Design review of the part built by this model. Coordinates are the model's own, in mm. Round coordinates to 2 decimals unless told otherwise and drop trailing zeros. Order: outer loops, then holes, each group sorted by start corner. A loop starts at its lowest first (then second) coordinate and runs counter-clockwise, first axis right, second up. Notation, with made-up numbers: M 14,33 L 64,33 A38 cw 64,72 Z; hole C -37,-36 d8. An arc over 180 degrees is marked long. Use a Markdown table: item, result. Add a question column.
(1) Take a section at B-B (z = -36.5). Write out the cut boundary in (x, y).
(2) For pin 1 (1.5 mm diameter, centred on y = -1, z = 7, fed in from +X); pin 2 (23 mm diameter, centred on x = 75.01, z = 0, fed in from -Y); pin 3 (2 mm diameter, centred on y = -3, z = -19, fed in from -X), all flat-tipped, find the tip position at first contact; note any pin that passes through.
(3) The part is to be moulded in two halves that separate along X. For faces 1 (the face through (-64.086, -3.131, 3.815)), 2 (the face through (1.22, -3.13, 63.49)), 3 (the face through (45, 0, 1)), say which applies: released by +X, released by -X, zero draft, split by the parting line, or undercut.
(4) Take a section at A-A (x = 85). Write out the cut boundary in (y, z).
(5) Take a section at C-C (z = 9). Write out the cut boundary in (x, y).
(6) To check wall thickness, follow probe 1 along Z at (x, y) = (0, -2.5); probe 2 along X at (y, z) = (-4.25, 4); probe 3 along Z at (x, y) = (74.5, -1.25). State the ranges of each line that lie inside material, in increasing order. Write a range as from..to.
(7) Take a section at D-D (y = -2). Write out the cut boundary in (x, z).
```python
from build123d import *

# Parameters (mm, degrees)
F0_R     = 12.7
F1_DEPTH = 6.35


# Not quite as in the source:
# - a length typed as a fraction of an inch, garbled in the dataset ("3 / 203.2 mm" for 3/8 in), is restored


with BuildPart() as f1:
    # F0 (on Front) → F1 (new body)
    with BuildSketch(Plane.XZ):
        with BuildLine():
            ThreePointArc((-46.13671875, -43.6308741946), (-24.8918341596, -58.4178619274), (0.4890866537, -63.4981164622))
            ThreePointArc((0.4890866537, -63.4981164622), (25.7887406506, -58.0275008566), (46.8033281156, -42.9150145905))
            ThreePointArc((46.8033281156, -42.9150145905), (59.5789989506, -33.7738186545), (74.9568035052, -30.5640903944))
            ThreePointArc((74.9568035052, -30.5640903944), (105.5782883644, 0), (74.9568035052, 30.5640903944))
            ThreePointArc((74.9568035052, 30.5640903944), (59.5789989506, 33.7738186545), (46.8033281156, 42.9150145905))
            ThreePointArc((46.8033281156, 42.9150145905), (0.4890866537, 63.4981164622), (-46.13671875, 43.6308741946))
            ThreePointArc((-46.13671875, 43.6308741946), (-59.3475236203, 34.5646316236), (-75.1176136364, 31.7315448688))
            ThreePointArc((-75.1176136364, 31.7315448688), (-107.95, 0), (-75.1176136364, -31.7315448688))
            ThreePointArc((-75.1176136364, -31.7315448688), (-59.3475236203, -34.5646316236), (-46.13671875, -43.6308741946))
        make_face()
        with Locations((-76.2, 0)):
            Circle(F0_R, mode=Mode.SUBTRACT)
        with BuildLine():
            ThreePointArc((0.3423606576, -44.4486815235), (-31.5517070159, 31.3096196781), (44.45, 0))
            ThreePointArc((44.45, 0), (31.5517070159, -31.3096196781), (0.3423606576, -44.4486815235))
        make_face(mode=Mode.SUBTRACT)
        with BuildLine():
            ThreePointArc((87.7141441822, 0), (83.9859725242, -8.9886759982), (74.9903180088, -12.6999776501))
            ThreePointArc((74.9903180088, -12.6999776501), (66.0423158402, 8.9886759982), (87.7141441822, 0))
        make_face(mode=Mode.SUBTRACT)
    extrude(amount=F1_DEPTH)


solid = f1.part
```
Verdict:
| question | item | result |
|---|---|---|
| 1 | outline | M -55.32,-6.35 L -25.37,-6.35 L -25.37,0 L -55.32,0 Z; M 25.37,-6.35 L 54.46,-6.35 L 54.46,0 L 25.37,0 Z |
| 2 | pin 1 | stops at x = 104.93 |
| 2 | pin 2 | passes through |
| 2 | pin 3 | stops at x = -102.35 |
| 3 | face 1 | undercut |
| 3 | face 2 | split by the parting line |
| 3 | face 3 | zero draft |
| 4 | outline | M -6.35,-28.89 L 0,-28.89 L 0,-7.85 L -6.35,-7.85 Z; M -6.35,7.85 L 0,7.85 L 0,28.89 L -6.35,28.89 Z |
| 5 | outline | M -106.65,-6.35 L -85.16,-6.35 L -85.16,0 L -106.65,0 Z; M -67.24,-6.35 L -43.53,-6.35 L -43.53,0 L -67.24,0 Z; M 43.53,-6.35 L 66.05,-6.35 L 66.05,0 L 43.53,0 Z; M 83.97,-6.35 L 104.22,-6.35 L 104.22,0 L 83.97,0 Z |
| 6 | probe 1 | z = -63.5..-44.45, 44.45..63.5 |
| 6 | probe 2 | x = -107.7..-88.25, -64.15..-44.27, 44.27..62.96, 87.07..105.32 |
| 6 | probe 3 | z = -30.57..-12.69, 12.69..30.57 |
| 7 | outline | M -75.12,-31.73 A38.1 cw -46.14,-43.63 A63.5 ccw 46.8,-42.92 A38.1 cw 74.96,-30.56 A30.56 ccw 74.96,30.56 A38.1 cw 46.8,42.92 A63.5 ccw -46.14,43.63 A38.1 cw -75.12,31.73 A31.75 ccw long Z; hole C -76.2,0 d25.4; hole C 0,0 d88.9; hole C 75.01,0 d25.4 |
